Source: CAD feature listing. Evaluate the final solid. Frame: model axes, mm. Face numbers are marked on the shaded views. A direction names the side the tool comes from. Give positions to 0.01 mm unless a question says otherwise; leave off trailing zeros. Loops run counter-clockwise (first coordinate to the right, second up) from the corner with the lowest first, then second, coordinate; pieces in that order, holes last. Notation, with made-up numbers: (47.5, 89) -> (58.5, 89) arc R27 ccw to (58.5, 118) -> close; hole circle Ø9 at (71.25, 29.25). An arc over 180 degrees is marked (long way). Return JSON: item names as keys, results as strings. Group by question number.
(1) Access query for the marked faces 1, 2 and 3. Directions: +Z, -Z, +X, -X, +Y, -Y. A direction counts if a zero-diameter tool reaches every point of the face in a straight line with its end or side. Return the directions, or none.
(2) Ray query, line 1 (Y direction, x = 3.5, z = 12) (3 decimals); line 2 (Y direction, x = 0, z = 8.5) (1 decimal). Return the intervals inside material, ascending. Write a range as from..to.
(3) Cut plane A-A on z = 10. Return loops of the section in (x, y) (3 decimals).
(4) Pin query (flat end, axial travel): pin 1 (1.5 mm diameter, centred on y = 5, z = 6.5, fed in from -X); pin 2 (8 mm diameter, centred on x = 5, y = -5, fed in from -Z); pin 3 (7.5 mm diameter, centred on x = 0, y = 0, fed in from +Z); pin 4 (6 mm diameter, centred on x = -2.5, y = 7.5, fed in from -Z) (3 decimals). Return the tip coordinate at first contact, or that it passes through.
(5) Cut plane B-B on x = 0. Return loops of the section in (y, z) (1 decimal).
(6) Draft query along Y for the marked faces 4, 5 and 6. Return one class per face: released by +Y, released by -Y, zero draft, split by the parting line, or undercut.
(7) Cut plane D-D on y = 5.75. Return loops of the section in (x, z) (1 decimal), then the cut area to 3 significant figures.
```python
from build123d import *

# Parameters (mm, degrees)
F0_R     = 4.7625
F1_DEPTH = 17.4625
F3_W     = 19.05
F3_H     = 7.9375
F4_DEPTH = 9.525
F6_DEPTH = 6.35
F2_R     = 3.175
F7_DEPTH = 17.4625


with BuildPart() as f1:
    # F0 (on Top) → F1 (new body)
    with BuildSketch(Plane.XY):
        Circle(F0_R)
    extrude(amount=F1_DEPTH)

    # F3 (on Front) → F4 (join, symmetric)
    with BuildSketch(Plane.XZ):
        with Locations((0, 13.49375)):
            Rectangle(F3_W, F3_H)
    extrude(amount=F4_DEPTH, both=True)

    # F5 (on face) → F6 (cut)
    with BuildSketch(Plane.XY.offset(17.4625)):
        with BuildLine():
            Line((6.985, 8.255), (-6.985, 8.255))
            ThreePointArc((-6.985, 8.255), (-7.883026, 7.883026), (-8.255, 6.985))
            Line((-8.255, 6.985), (-8.255, -6.985))
            ThreePointArc((-8.255, -6.985), (-7.883026, -7.883026), (-6.985, -8.255))
            Line((-6.985, -8.255), (6.985, -8.255))
            ThreePointArc((6.985, -8.255), (7.883026, -7.883026), (8.255, -6.985))
            Line((8.255, -6.985), (8.255, 6.985))
            ThreePointArc((8.255, 6.985), (7.883026, 7.883026), (6.985, 8.255))
        make_face()
    extrude(amount=-F6_DEPTH, mode=Mode.SUBTRACT)

    # F2 (on face) → F7 (cut)
    with BuildSketch(Plane.XY):
        Circle(F2_R)
    extrude(amount=F7_DEPTH, mode=Mode.SUBTRACT)


solid = f1.part
```
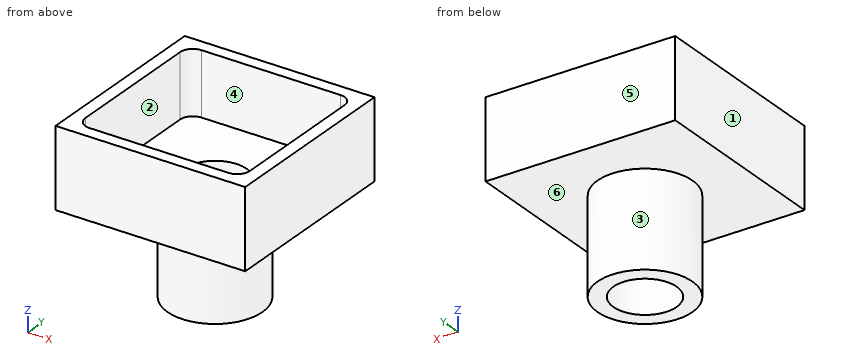
Answers:
{
 "1": {"face 1": "+Z, -Z, -X, +Y, -Y", "face 2": "+Z", "face 3": "-Z"},
 "2": {"line 1": "-9.525..-8.255, 8.255..9.525", "line 2": "-4.8..-3.2, 3.2..4.8"},
 "3": {"outline": "(-9.525, -9.525) -> (9.525, -9.525) -> (9.525, 9.525) -> (-9.525, 9.525) -> close; hole circle Ø6.35 at (0, 0)"},
 "4": {"pin 1": "x = -2.15", "pin 2": "z = 0", "pin 3": "z = 11.11", "pin 4": "z = 9.525"},
 "5": {"outline": "(-9.5, 9.5) -> (-4.8, 9.5) -> (-4.8, 0) -> (-3.2, 0) -> (-3.2, 11.1) -> (-8.3, 11.1) -> (-8.3, 17.5) -> (-9.5, 17.5) -> close; (3.2, 0) -> (4.8, 0) -> (4.8, 9.5) -> (9.5, 9.5) -> (9.5, 17.5) -> (8.3, 17.5) -> (8.3, 11.1) -> (3.2, 11.1) -> close"},
 "6": {"face 4": "undercut", "face 5": "released by +Y", "face 6": "zero draft"},
 "7": {"outline": "(-9.5, 9.5) -> (9.5, 9.5) -> (9.5, 17.5) -> (8.3, 17.5) -> (8.3, 11.1) -> (-8.3, 11.1) -> (-8.3, 17.5) -> (-9.5, 17.5) -> close", "area": "46.4 mm²"}
}
